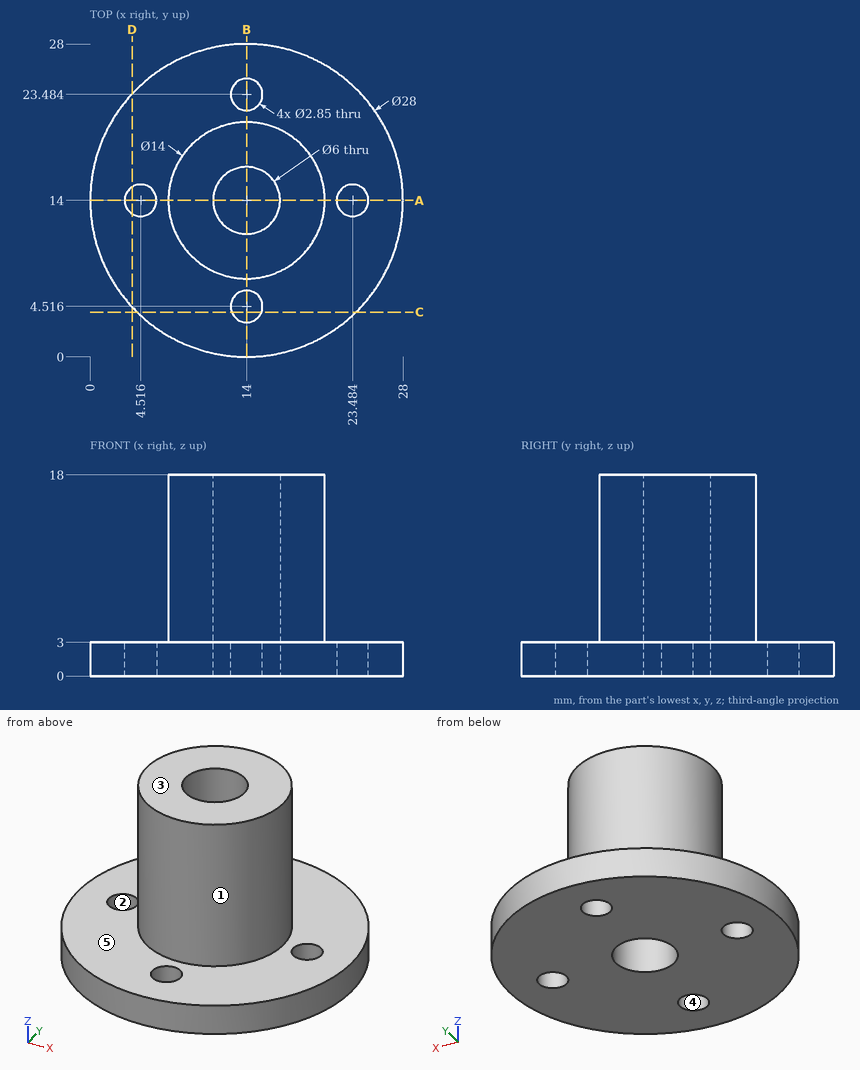
The drawing under review shows one solid part. Ordinate dimensions are in mm from its lowest x, y, z. A direction names the side the tool comes from. Round coordinates to 2 decimals unless told otherwise and drop trailing zeros. Order: outer loops, then holes, each group sorted by start corner. A loop starts at its lowest first (then second) coordinate and runs counter-clockwise, first axis right, second up. Notation, with made-up numbers: (-2, -38) -> (50, -38) arc R19 ccw to (50, -15) -> close; hole circle Ø2 at (30.25, 52.5). An arc over 180 degrees is marked (long way). Return JSON: item names as keys, results as strings.
1. Take a section at C-C (y = 4). Write out the cut boundary in (x, z), then the cut area to 3 significant figures.
Answer block:
{"outline": "(4.2, 0) -> (12.67, 0) -> (12.67, 3) -> (4.2, 3) -> close; (15.33, 0) -> (23.8, 0) -> (23.8, 3) -> (15.33, 3) -> close", "area": "50.8 mm²"}
2. Take a section at D-D (x = 3.75). Write out the cut boundary in (y, z), then the cut area to 3 significant figures.
Answer block:
{"outline": "(4.46, 0) -> (12.8, 0) -> (12.8, 3) -> (4.46, 3) -> close; (15.2, 0) -> (23.54, 0) -> (23.54, 3) -> (15.2, 3) -> close", "area": "50.0 mm²"}
3. For the marked faces 4 and 5, list the 3-axis set-ups (+Z, -Z, +X, -X, +Y, -Y) from which the entire face can be reached by the end or side of a thin tool; tool diameter is ignored.
Answer block:
{"face 4": "+Z, -Z", "face 5": "+Z"}
4. Insertion check: P1, Ø9.5, axis at x = 14, y = 14, coming from the +Z side; P2, Ø4.5, axis at x = 14, y = 23.48, coming from the +Z side; P3, Ø1.5, axis at y = 12.5, z = 13.5, coming from the -X side; P4, Ø1, axis at x = 19.5, z = 8, coming from the -Y side. Each pin has a flat end and moves straight along its axis. Give the tip position at first contact, or say it passes through.
Answer block:
{"P1": "stops at z = 18", "P2": "stops at z = 3", "P3": "stops at x = 7.04", "P4": "stops at y = 9.1"}
5. Take a section at A-A (y = 14). Write out the cut boundary in (x, z).
Answer block:
{"outline": "(0, 0) -> (3.09, 0) -> (3.09, 3) -> (0, 3) -> close; (5.94, 0) -> (11, 0) -> (11, 18) -> (7, 18) -> (7, 3) -> (5.94, 3) -> close; (17, 0) -> (22.06, 0) -> (22.06, 3) -> (21, 3) -> (21, 18) -> (17, 18) -> close; (24.91, 0) -> (28, 0) -> (28, 3) -> (24.91, 3) -> close"}
6. For L1, parallel to Y at x = 14, z = 13.75; L2, parallel to Z at x = 11.75, y = 26.25; L3, parallel to X at y = 15.75, z = 8.5, list the stretches that pass through material, from the lowest coordinate up. Write a range as [from, to].
Answer block:
{"L1": "y = [7, 11], [17, 21]", "L2": "z = [0, 3]", "L3": "x = [7.22, 11.56], [16.44, 20.78]"}
7. The part is to be moulded in two halves that separate along Y. For the marked faces 1, 2 and 3, say which applies: +Y half, -Y half, draft (parallel to the pull), parting line (faces both ways), or undercut.
Answer block:
{"face 1": "parting line", "face 2": "undercut", "face 3": "draft"}
